from build123d import *

# Parameters (mm, degrees)
SKETCH1_W           = 28
SKETCH1_H           = 28
BOSS_EXTRUDE1_DEPTH = 35
SKETCH2_R           = 14
BOSS_EXTRUDE2_DEPTH = 35
SKETCH3_R           = 9
BOSS_EXTRUDE3_DEPTH = 2
SKETCH4_R           = 3
BOSS_EXTRUDE4_DEPTH = 16
CUT_EXTRUDE1_START  = -12
CUT_EXTRUDE1_DEPTH  = 12
SKETCH6_R           = 1.5
CUT_EXTRUDE2_DEPTH  = 2
SKETCH7_R           = 2.5
BOSS_EXTRUDE5_DEPTH = 9.5
CHAMFER1_SIZE       = 2
SKETCH8_R           = 1.5
CUT_EXTRUDE3_DEPTH  = 5


with BuildPart() as part:
    # Sketch1 → Boss-Extrude1 (new body)
    with BuildSketch(Plane.XY):
        Rectangle(SKETCH1_W, SKETCH1_H)
    extrude(amount=BOSS_EXTRUDE1_DEPTH)

    # Sketch2 → Boss-Extrude2 (add)
    with BuildSketch(Plane.XY.offset(35)):
        Circle(SKETCH2_R)
    extrude(amount=BOSS_EXTRUDE2_DEPTH)

    # Sketch3 → Boss-Extrude3 (add)
    with BuildSketch(Plane.XY.offset(70)):
        Circle(SKETCH3_R)
    extrude(amount=BOSS_EXTRUDE3_DEPTH)

    # Sketch4 → Boss-Extrude4 (add)
    with BuildSketch(Plane.XY.offset(72)):
        Circle(SKETCH4_R)
    extrude(amount=BOSS_EXTRUDE4_DEPTH)

    # Sketch5 → Cut-Extrude1 (cut)
    with BuildSketch(Plane.XY.offset(88).offset(CUT_EXTRUDE1_START)):
        with BuildLine():
            Line((-2.236067977, 2), (2.236067977, 2))
            ThreePointArc((2.236067977, 2), (0, 3), (-2.236067977, 2))
        make_face()
    extrude(amount=CUT_EXTRUDE1_DEPTH, mode=Mode.SUBTRACT)

    # Sketch6 → Cut-Extrude2 (cut)
    with BuildSketch(Plane(origin=(0, 0, 0), x_dir=(-1, 0, 0), z_dir=(0, 0, -1))):
        with Locations((9.5, 0)):
            Circle(SKETCH6_R)
        with Locations(Location((-9.5, 0, 0), (0, 0, 180))):
            Circle(SKETCH6_R)
    extrude(amount=-CUT_EXTRUDE2_DEPTH, mode=Mode.SUBTRACT)

    # Sketch7 → Boss-Extrude5 (add)
    with BuildSketch(Plane(origin=(0, 0, 0), x_dir=(-1, 0, 0), z_dir=(0, 0, -1))):
        Circle(SKETCH7_R)
    extrude(amount=BOSS_EXTRUDE5_DEPTH)

    # Chamfer1
    chamfer1_edges = [part.edges().sort_by_distance(p)[0] for p in [
        (14, -14, 17.5),
        (-14, -14, 17.5),
        (-14, 14, 17.5),
        (14, 14, 17.5),
    ]]
    chamfer(chamfer1_edges, length=CHAMFER1_SIZE)

    # Sketch8 → Cut-Extrude3 (cut)
    with BuildSketch(Plane.XY.offset(70)):
        with Locations((0, 11)):
            Circle(SKETCH8_R)
        with Locations((11, 0)):
            Circle(SKETCH8_R)
        with Locations((0, -11)):
            Circle(SKETCH8_R)
        with Locations((-11, 0)):
            Circle(SKETCH8_R)
    extrude(amount=-CUT_EXTRUDE3_DEPTH, mode=Mode.SUBTRACT)


solid = part.part
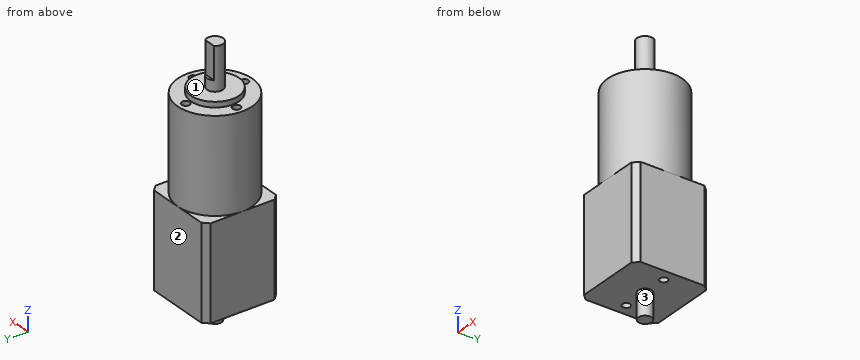
Work out the finished part from the listing and answer in its coordinate system (mm). Face numbers are marked on the shaded views. A direction names the side the tool comes from. Coordinates: 2 decimals unless noted, no trailing zeros. Loops run counter-clockwise (first coordinate to the right, second up) from the corner with the lowest first, then second, coordinate; pieces in that order, holes last. Notation, with made-up numbers: M 81,-8.75 L 117,-8.75 A14 cw 117,4.25 Z; hole C 46,46.25 d5. An arc over 180 degrees is marked long. Answer in a Markdown table with one row per item. Add a question column.
1. Flat-ended cylindrical pins translate along their axes: P1, Ø5, axis at x = 9.5, y = -3, coming from the +Z side; P2, Ø3, axis at y = -9, z = 46.5, coming from the +X side; P3, Ø1.5, axis at y = 2, z = 59, coming from the -X side; P4, Ø14, axis at x = -5.5, y = -2, coming from the +Z side. Find the tip coordinate at first contact, or state that the pin passes through.
2. Find section C-C, the plane x = 5.5. Write down the section's boundary in (y, z), then the cut area to 3 significant figures.
3. Find section A-A, the plane y = 11. Write down the section's boundary in (x, z), then the cut area to 3 significant figures.
4. Consider L1, parallel to Y at x = -9.5, z = 0.4; L2, parallel to Z at x = -6, y = -9.25; L3, parallel to Z at x = 7.5, y = -12. Determine where each line is inside the solid, lowest interval first.
5. A tool of negligible diameter and unlimited length cuts with its end or side. For the marked faces 1, 2 and 3, from which of +Z, -Z, +X, -X, +Y, -Y can it reach the whole face along a straight path? Write none if from no direction.
6. Find section B-B, the plane z = 78. Write down the section's boundary in (x, y).
7. Find section D-D, the plane z = 37.5. Write down the section's boundary in (x, y), then the cut area to 3 significant figures.
Reported:
| question | item | result |
|---|---|---|
| 1 | P1 | stops at z = 72 |
| 1 | P2 | stops at x = 11.82 |
| 1 | P3 | stops at x = -13.94 |
| 1 | P4 | stops at z = 88 |
| 2 | outline | M -14,0 L 14,0 L 14,35 L 12.87,35 L 12.87,70 L 7.12,70 L 7.12,72 L -7.12,72 L -7.12,70 L -12.87,70 L -12.87,35 L -14,35 Z |
| 2 | area | 1,910 mm^2 |
| 3 | outline | M -14,0 L 14,0 L 14,35 L 8.66,35 L 8.66,70 L 1.5,70 L 1.5,65 L -1.5,65 L -1.5,70 L -8.66,70 L -8.66,35 L -14,35 Z |
| 3 | area | 1,570 mm^2 |
| 4 | L1 | y = -14 to -1.5, 1.5 to 14 |
| 4 | L2 | z = 0 to 70 |
| 4 | L3 | z = 0 to 35 |
| 5 | face 1 | +Z |
| 5 | face 2 | +Z, -Z, +X, -X, +Y |
| 5 | face 3 | -Z |
| 6 | outline | M -2.24,2 A3 ccw long 2.24,2 Z |
| 7 | outline | C 0,0 d28 |
| 7 | area | 616 mm^2 |
